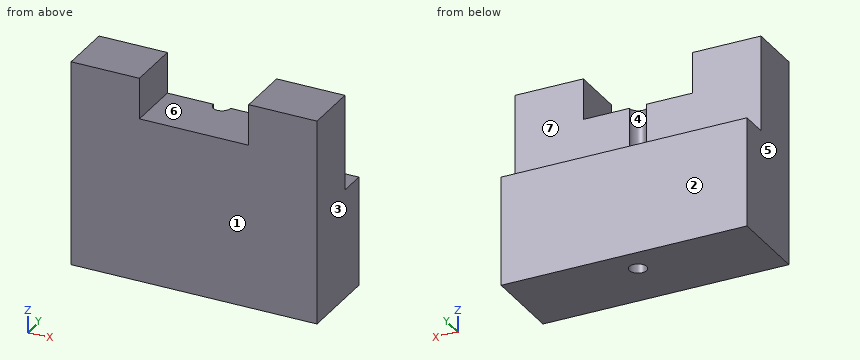
```python
from build123d import *

# Parameters (mm, degrees)
SKETCH2_W           = 18
SKETCH2_H           = 15
BOSS_EXTRUDE2_DEPTH = 6
CUT_EXTRUDE3_DEPTH  = 2
SKETCH7_W           = 8
SKETCH7_H           = 3
CUT_EXTRUDE4_DEPTH  = 24.769728648
SKETCH12_R          = 0.635
CUT_EXTRUDE5_DEPTH  = 25.186773245


with BuildPart() as part:
    # Sketch2 → Boss-Extrude2 (new body)
    with BuildSketch(Plane(origin=(0, 0, 0), x_dir=(1, 0, 0), z_dir=(0, 1, 0))):
        with Locations((-9, 7.5)):
            Rectangle(SKETCH2_W, SKETCH2_H)
    extrude(amount=BOSS_EXTRUDE2_DEPTH)

    # Sketch6 → Cut-Extrude3 (cut)
    with BuildSketch(Plane(origin=(0, 6, 0), x_dir=(1, 0, 0), z_dir=(0, 1, 0))):
        Polygon((0, 7), (0, 0), (-2, 0), (-18, 0), (-18, 7), (-2, 7), align=None)
    extrude(amount=-CUT_EXTRUDE3_DEPTH, mode=Mode.SUBTRACT)

    # Sketch7 → Cut-Extrude4 (cut, through all)
    with BuildSketch(Plane(origin=(0, 4, 0), x_dir=(1, 0, 0), z_dir=(0, 1, 0))):
        with Locations((-9, 1.5)):
            Rectangle(SKETCH7_W, SKETCH7_H)
    extrude(amount=-CUT_EXTRUDE4_DEPTH, mode=Mode.SUBTRACT)

    # Sketch12 → Cut-Extrude5 (cut, through all)
    with BuildSketch(Plane(origin=(0, 0, -15), x_dir=(-1, 0, 0), z_dir=(0, 0, -1))):
        with Locations((9, 4)):
            Circle(SKETCH12_R)
    extrude(amount=-CUT_EXTRUDE5_DEPTH, mode=Mode.SUBTRACT)


solid = part.part
```
Verification items for the finished model (mm, model axes). Face numbers are marked on the shaded views. A direction names the side the tool comes from. Coordinates: 2 decimals unless noted, no trailing zeros. Loops run counter-clockwise (first coordinate to the right, second up) from the corner with the lowest first, then second, coordinate; pieces in that order, holes last. Notation, with made-up numbers: (28.25, -11.5) - (43.25, -11.5) arc R19 cw to (43.25, 17.5) - close; hole circle Ø9 at (44, -16). An arc over 180 degrees is marked (long way). Answer as a JSON object with one key per item and string values.
(1) Access from +Z, -Z, +X, -X, +Y, -Y to the whole of each face (thin tool, end or side, straight path). Record for the marked faces 5, 6 and 7.
Response:
{"face 5": "+Z, -Z, -X, +Y, -Y", "face 6": "+Z, +Y, -Y", "face 7": "+Z, +X, -X, +Y"}
(2) Cross-section at D-D, the plane x = -16.5. Record the boundary of the cut face in (y, z), then the cut area to 3 significant figures.
Response:
{"outline": "(0, -15) - (6, -15) - (6, -7) - (4, -7) - (4, 0) - (0, 0) - close", "area": "76.0 mm²"}
(3) Cross-section at A-A, the plane x = -9. Record the boundary of the cut face in (y, z) (3 decimals).
Response:
{"outline": "(0, -15) - (3.365, -15) - (3.365, -3) - (0, -3) - close; (4.635, -15) - (6, -15) - (6, -7) - (4.635, -7) - close"}
(4) Scan lines: line 1 along Y through (x, z) = (-9, -7.5) (3 decimals); line 2 along X through (y, z) = (4, -11) (3 decimals); line 3 along Z through (x, y) = (-3, 4.3). Record each from-to range of solid material in increasing order.
Response:
{"line 1": "y = 0 to 3.365, 4.635 to 6", "line 2": "x = -18 to -9.635, -8.365 to 0", "line 3": "z = -15 to -7"}
(5) Cross-section at B-B, the plane y = 1.65. Record the boundary of the cut face in (x, z), then the cut area to 3 significant figures.
Response:
{"outline": "(-18, -15) - (0, -15) - (0, 0) - (-5, 0) - (-5, -3) - (-13, -3) - (-13, 0) - (-18, 0) - close", "area": "246 mm²"}
(6) Go/stop test with flat-tipped pins: pin 1 Ø0.8 at (x, y) = (-9, 4) entering from +Z; pin 2 Ø2 at (x, z) = (-15.5, -3) entering from +Y; pin 3 Ø0.6 at (x, y) = (-6.5, 5) entering from +Z; pin 4 Ø1 at (x, y) = (-15.5, 1) entering from +Z. Record where each tip stops, or that it passes through.
Response:
{"pin 1": "passes through", "pin 2": "stops at y = 4", "pin 3": "stops at z = -7", "pin 4": "stops at z = 0"}
(7) Mould release check, pull along Y, two halves, no side actions. Record for the marked faces 1, 2, 3 and 4: pulls with the +Y half, pulls with the -Y half, needs draft (parallel to the pull), parting line crosses it, or undercut.
Response:
{"face 1": "pulls with the -Y half", "face 2": "pulls with the +Y half", "face 3": "needs draft", "face 4": "undercut"}
(8) Cross-section at C-C, the plane z = -4.5. Record the boundary of the cut face in (x, y) (3 decimals).
Response:
{"outline": "(-18, 0) - (0, 0) - (0, 4) - (-8.365, 4) arc R0.635 cw to (-9.635, 4) - (-18, 4) - close"}
